```python
from build123d import *

# Parameters (mm, degrees)
SKETCH1_R           = 5
SKETCH1_R_2         = 3
BOSS_EXTRUDE1_DEPTH = 10
SKETCH2_R           = 12.5
BOSS_EXTRUDE2_DEPTH = 5
SKETCH6_R           = 1.5
CUT_EXTRUDE1_DEPTH  = 5
SKETCH7_R           = 1.5
CUT_EXTRUDE2_DEPTH  = 5
SKETCH8_R           = 3
CUT_EXTRUDE3_DEPTH  = 5


with BuildPart() as part:
    # Sketch1 → Boss-Extrude1 (new body)
    with BuildSketch(Plane(origin=(0, 0, 0), x_dir=(1, 0, 0), z_dir=(0, 1, 0))):
        with Locations(Location((0, 0, 0), (0, 0, 270))):
            Circle(SKETCH1_R)
        with Locations(Location((0, 0, 0), (0, 0, 270))):
            Circle(SKETCH1_R_2, mode=Mode.SUBTRACT)
    extrude(amount=-BOSS_EXTRUDE1_DEPTH)

    # Sketch2 → Boss-Extrude2 (add)
    with BuildSketch(Plane.XZ.offset(10)):
        with Locations(Location((0, 0, 0), (0, 0, 270))):
            Circle(SKETCH2_R)
    extrude(amount=BOSS_EXTRUDE2_DEPTH)

    # Sketch6 → Cut-Extrude1 (cut)
    with BuildSketch(Plane(origin=(0, -10, 0), x_dir=(1, 0, 0), z_dir=(0, 1, 0))):
        with Locations(Location((0, 8.75, 0), (0, 0, 270))):
            Circle(SKETCH6_R)
        with Locations(Location((8.75, 0, 0), (0, 0, 270))):
            Circle(SKETCH6_R)
        with Locations(Location((0, -8.75, 0), (0, 0, 270))):
            Circle(SKETCH6_R)
        with Locations(Location((-8.75, 0, 0), (0, 0, 270))):
            Circle(SKETCH6_R)
    extrude(amount=-CUT_EXTRUDE1_DEPTH, mode=Mode.SUBTRACT)

    # Sketch7 → Cut-Extrude2 (cut)
    with BuildSketch(Plane(origin=(0, 0, -5), x_dir=(-1, 0, 0), z_dir=(0, 0, -1))):
        with Locations((0, -5)):
            Circle(SKETCH7_R)
    extrude(amount=-CUT_EXTRUDE2_DEPTH, mode=Mode.SUBTRACT)

    # Sketch8 → Cut-Extrude3 (cut)
    with BuildSketch(Plane(origin=(0, -10, 0), x_dir=(1, 0, 0), z_dir=(0, 1, 0))):
        with Locations(Location((0, 0, 0), (0, 0, 270))):
            Circle(SKETCH8_R)
    extrude(amount=-CUT_EXTRUDE3_DEPTH, mode=Mode.SUBTRACT)


solid = part.part
```
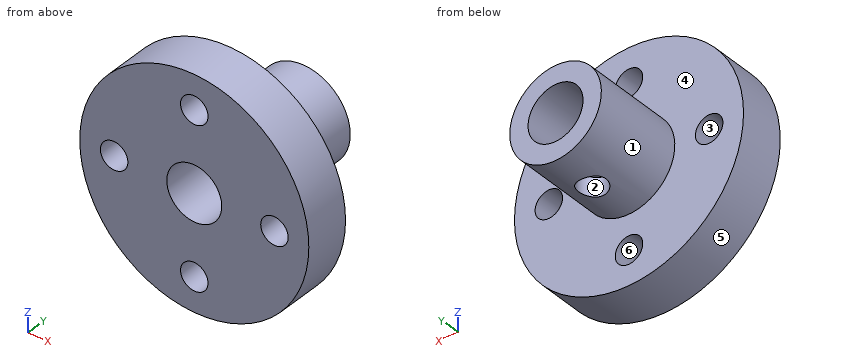
The model under review builds one solid part; all positions refer to its coordinate system, in mm. Face numbers are marked on the shaded views. A direction names the side the tool comes from. Coordinates: 2 decimals unless noted, no trailing zeros. Write each loop counter-clockwise with the first axis right and the second up, starting at its lowest first coordinate (ties: lowest second). Pieces come first, ordered by that corner, then holes. Notation, with made-up numbers: (42.5, -16.75) - (97.5, -16.75) arc R28 cw to (97.5, 5.25) - close; hole circle Ø3 at (-31, 20). An arc over 180 degrees is marked (long way). Answer in a Markdown table with one row per item. Add a question column.
Q1. Clearance check with flat-ended pins moving along their axes: pin 1 (2.5 mm diameter, centred on x = 8.75, z = 0, fed in from +Y); pin 2 (1 mm diameter, centred on y = -13.5, z = 1, fed in from +X); pin 3 (3.5 mm diameter, centred on x = 0, y = -5, fed in from -Z); pin 4 (1 mm diameter, centred on y = -3.5, z = 2.5, fed in from +X). State where each tip first meets the part, or that it passes through.
Q2. Draft analysis for pull direction Z (two halves, no side actions). For the marked faces 4, 5 and 6, state which applies: +Z half, -Z half, draft (parallel to the pull), parting line (faces both ways), or undercut.
Q3. To check wall thickness, follow line 1 along X through (y, z) = (-14, 0); line 2 along Z through (x, y) = (1, -10.25); line 3 along X through (y, z) = (-13.5, 1.75). State the ranges of each line that lie inside material, in increasing order. Write a range as from..to.
Q4. Consider section C-C on z = 8.75. Give the boundary of the cut face in (x, y).
Q5. Consider section D-D on y = -13.5. Give the boundary of the cut face in (x, z).
Q6. Consider section B-B on x = 0. Give the boundary of the cut face in (y, z).
Q7. For the marked faces 1, 2 and 3, list the 3-axis set-ups (+Z, -Z, +X, -X, +Y, -Y) from which the entire face can be reached by the end or side of a thin tool; tool diameter is ignored.
Q8. Consider section A-A on z = 0. Give the boundary of the cut face in (x, y).
Answers below:
| question | item | result |
|---|---|---|
| 1 | pin 1 | through |
| 1 | pin 2 | x = 12.49 |
| 1 | pin 3 | z = -5 |
| 1 | pin 4 | x = 4.58 |
| 2 | face 4 | draft |
| 2 | face 5 | parting line |
| 2 | face 6 | undercut |
| 3 | line 1 | -12.5..-10.25, -7.25..-3, 3..7.25, 10.25..12.5 |
| 3 | line 2 | -12.46..-9.87, -7.63..-2.83, 2.83..7.63, 9.87..12.46 |
| 3 | line 3 | -12.38..-2.44, 2.44..12.38 |
| 4 | outline | (-8.93, -15) - (-1.5, -15) - (-1.5, -10) - (-8.93, -10) - close; (1.5, -15) - (8.93, -15) - (8.93, -10) - (1.5, -10) - close |
| 5 | outline | circle Ø25 at (0, 0); hole circle Ø3 at (-8.75, 0); hole circle Ø6 at (0, 0); hole circle Ø3 at (0, -8.75); hole circle Ø3 at (0, 8.75); hole circle Ø3 at (8.75, 0) |
| 6 | outline | (-15, -12.5) - (-10, -12.5) - (-10, -10.25) - (-15, -10.25) - close; (-15, -7.25) - (-10, -7.25) - (-10, -5) - (-6.5, -5) - (-6.5, -3) - (-15, -3) - close; (-15, 3) - (0, 3) - (0, 5) - (-10, 5) - (-10, 7.25) - (-15, 7.25) - close; (-15, 10.25) - (-10, 10.25) - (-10, 12.5) - (-15, 12.5) - close; (-3.5, -5) - (0, -5) - (0, -3) - (-3.5, -3) - close |
| 7 | face 1 | +Y |
| 7 | face 2 | -Z |
| 7 | face 3 | +Y, -Y |
| 8 | outline | (-12.5, -15) - (-10.25, -15) - (-10.25, -10) - (-12.5, -10) - close; (-7.25, -15) - (-3, -15) - (-3, 0) - (-5, 0) - (-5, -10) - (-7.25, -10) - close; (3, -15) - (7.25, -15) - (7.25, -10) - (5, -10) - (5, 0) - (3, 0) - close; (10.25, -15) - (12.5, -15) - (12.5, -10) - (10.25, -10) - close |
